```python
from build123d import *

# Parameters (mm, degrees)
ESQUISSE1_W             = 7.5
ESQUISSE1_H             = 3.75
BOSS_EXTRU_1_DEPTH      = 7.5
BOSS_EXTRU_1_2_DEPTH    = 7.5
ESQUISSE2_R             = 2.25
ENL_V_MAT_EXTRU_1_DEPTH = 58.737772997
ESQUISSE4_W             = 31.7
ESQUISSE4_H             = 43.35
BOSS_EXTRU_2_DEPTH      = 2
ESQUISSE5_W             = 34.15
ESQUISSE5_H             = 46.15
BOSS_EXTRU_3_DEPTH      = 3


with BuildPart() as part:
    # Esquisse1 → Boss.-Extru.1 (new body)
    with BuildSketch(Plane.XY):
        with Locations((6.831943462, 26.473190482)):
            Rectangle(ESQUISSE1_W, ESQUISSE1_H)
    extrude(amount=BOSS_EXTRU_1_DEPTH)


with BuildPart() as body_2:
    # Esquisse1 → Boss.-Extru.1 2 (new body)
    with BuildSketch(Plane.XY):
        with Locations((6.831943462, -27.514582515)):
            Rectangle(ESQUISSE1_W, ESQUISSE1_H)
    extrude(amount=BOSS_EXTRU_1_2_DEPTH)


with BuildPart() as enl_v_mat_extru_1_tool:
    # Esquisse2 → Enlèv. mat.-Extru.1 (new body, through all)
    with BuildSketch(Plane(origin=(0, 28.348190482, 0), x_dir=(1, 0, 0), z_dir=(0, 1, 0))):
        with Locations((6.831943462, -3.75)):
            Circle(ESQUISSE2_R)
    extrude(amount=-ENL_V_MAT_EXTRU_1_DEPTH)


with BuildPart() as part_1:
    add(part.part)

    # Enlèv. mat.-Extru.1: cut by enl_v_mat_extru_1_tool
    add(enl_v_mat_extru_1_tool.part, mode=Mode.SUBTRACT)



with BuildPart() as body_2_1:
    add(body_2.part)

    # Enlèv. mat.-Extru.1: cut by enl_v_mat_extru_1_tool
    add(enl_v_mat_extru_1_tool.part, mode=Mode.SUBTRACT)


with BuildPart() as part_2:
    add(part_1.part)

    add(body_2_1.part)  # Boss.-Extru.2 merges body 2
    # Esquisse4 → Boss.-Extru.2 (add)
    with BuildSketch(Plane.XY.offset(7.5)):
        Polygon((-15.243056538, 24.478190482), (-15.243056538, -25.521809518), (3.081943462, -29.389582515), (10.581943462, -29.389582515), (28.906943461, -25.521809518), (28.906943461, 24.478190482), (10.581943462, 28.348190482), (3.081943462, 28.348190482), align=None)
        with Locations((6.356943462, -0.426809518)):
            Rectangle(ESQUISSE4_W, ESQUISSE4_H, mode=Mode.SUBTRACT)
    extrude(amount=BOSS_EXTRU_2_DEPTH)

    # Esquisse5 → Boss.-Extru.3 (add)
    with BuildSketch(Plane.XY.offset(9.5)):
        Polygon((-15.243056538, 24.478190482), (3.081943462, 28.348190482), (10.581943462, 28.348190482), (28.906943461, 24.478190482), (28.906943461, -25.521809518), (10.581943462, -29.389582515), (3.081943462, -29.389582515), (-15.243056538, -25.521809518), align=None)
        with Locations((5.881943462, -0.331809518)):
            Rectangle(ESQUISSE5_W, ESQUISSE5_H, mode=Mode.SUBTRACT)
    extrude(amount=BOSS_EXTRU_3_DEPTH)


solid = part_2.part
```
Source: CAD feature listing. Evaluate the final solid. Frame: model axes, mm. A direction names the side the tool comes from. Coordinates: 2 decimals unless noted, no trailing zeros. Order: outer loops, then holes, each group sorted by start corner. A loop starts at its lowest first (then second) coordinate and runs counter-clockwise, first axis right, second up. Notation, with made-up numbers: M 18,13 L 75,13 A8 ccw 75,27 Z; hole C -9,-22.75 d8. An arc over 180 degrees is marked long. Write each question's results on one line, items separated by ' | '. Start each with the question number.
1) Access query for faces 1 (the face through (10.582, -28, 4)), 2 (the face through (6, -23.407, 11)), 3 (the face through (6, -22.102, 8)). Directions: +Z, -Z, +X, -X, +Y, -Y. A direction counts if a zero-diameter tool reaches every point of the face in a straight line with its end or side. Return the directions, or none.
2) Section query D-D (x = 21.5). Return the cut outline in (y, z), plus the area to 3 significant figures.
3) Draft query along X for faces 4 (the face through (19.87, -27.43, 9.96)), 5 (the face through (3.082, -28, 4)), 6 (the face through (6, 22.743, 11)), 7 (the face through (27, 0, 12.5)). Return one class per face: released by +X, released by -X, zero draft, split by the parting line, or undercut.
4) Section query B-B (y = -20). Return the cut outline in (x, z), plus the area to 3 significant figures.
5) Section query C-C (x = 8). Return the cut outline in (y, z).
6) Section query A-A (z = 3.75). Return the cut outline in (x, y), plus the area to 3 significant figures.
7) Line query: line 1 (X direction, y = 27.5, z = 3.75); line 2 (Y direction, x = 10, z = 2.5); line 3 (Z direction, x = -8, y = 24). Output: solid intervals per line, ascending. Write a range as from..to.
8) Contact query for flat-ended pins moving along their axis: pin 1 Ø3 at (y, z) = (-27, 3) entering from +X; pin 2 Ø22 at (x, y) = (10, -9) entering from -Z; pin 3 Ø6 at (x, z) = (16.5, 8.5) entering from +Y; pin 4 Ø1.6 at (x, z) = (13, 8) entering from -Y. Output: stop coordinate, or through.
Answers:
1) face 1: -Z, +X, +Y, -Y | face 2: +Z | face 3: +Z, -Z
2) outline: M -27.09,7.5 L -22.1,7.5 L -22.1,9.5 L -23.41,9.5 L -23.41,12.5 L -27.09,12.5 Z; M 21.25,7.5 L 26.04,7.5 L 26.04,12.5 L 22.74,12.5 L 22.74,9.5 L 21.25,9.5 Z | area: 40.5 mm^2
3) face 4: released by +X | face 5: released by -X | face 6: undercut | face 7: zero draft
4) outline: M -15.24,7.5 L -9.49,7.5 L -9.49,9.5 L -11.19,9.5 L -11.19,12.5 L -15.24,12.5 Z; M 22.21,7.5 L 28.91,7.5 L 28.91,12.5 L 22.96,12.5 L 22.96,9.5 L 22.21,9.5 Z | area: 54.9 mm^2
5) outline: M -29.39,0 L -25.64,0 L -25.64,1.83 L -29.39,1.83 Z; M -29.39,5.67 L -25.64,5.67 L -25.64,7.5 L -22.1,7.5 L -22.1,9.5 L -23.41,9.5 L -23.41,12.5 L -29.39,12.5 Z; M 21.25,7.5 L 24.6,7.5 L 24.6,5.67 L 28.35,5.67 L 28.35,12.5 L 22.74,12.5 L 22.74,9.5 L 21.25,9.5 Z; M 24.6,0 L 28.35,0 L 28.35,1.83 L 24.6,1.83 Z
6) outline: M 3.08,-29.39 L 4.58,-29.39 L 4.58,-25.64 L 3.08,-25.64 Z; M 3.08,24.6 L 4.58,24.6 L 4.58,28.35 L 3.08,28.35 Z; M 9.08,-29.39 L 10.58,-29.39 L 10.58,-25.64 L 9.08,-25.64 Z; M 9.08,24.6 L 10.58,24.6 L 10.58,28.35 L 9.08,28.35 Z | area: 22.5 mm^2
7) line 1: x = 3.08..4.58, 9.08..10.58 | line 2: y = -29.39..-25.64, 24.6..28.35 | line 3: z = 7.5..12.5
8) pin 1: stops at x = 10.58 | pin 2: passes through | pin 3: stops at y = 27.73 | pin 4: stops at y = -29.05
